Could you check a few things on this model? Use its own coordinates, in mm. Face numbers are marked on the shaded views. A direction names the side the tool comes from. Round coordinates to 2 decimals unless told otherwise and drop trailing zeros. Loops run counter-clockwise (first coordinate to the right, second up) from the corner with the lowest first, then second, coordinate; pieces in that order, holes last. Notation, with made-up numbers: (68.25, -12) -> (125.25, -12) arc R24 ccw to (125.25, 12) -> close; hole circle Ø10 at (68.5, -40). An arc over 180 degrees is marked (long way). One line per item, written item: value.
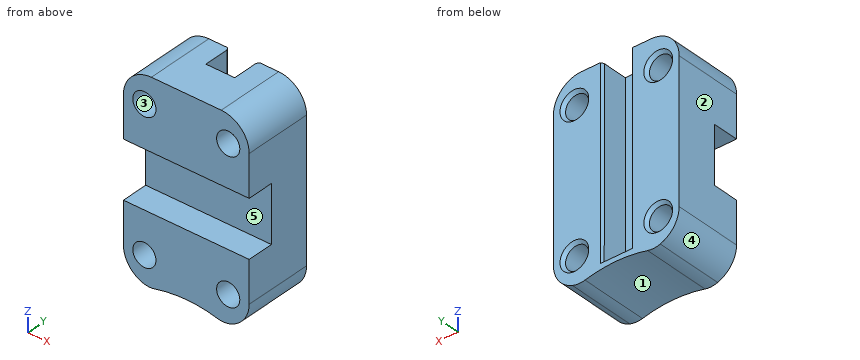
```python
from build123d import *

# Parameters (mm, degrees)
SKETCH1_W               = 45
SKETCH1_H               = 70
BOSS_EXTRUDE1_DEPTH     = 14.5
SKETCH2_W               = 20.25
SKETCH2_H               = 9.5
CUT_EXTRUDE1_DEPTH      = 1
CUT_EXTRUDE1_DEPTH_BACK = 46
SKETCH3_R               = 4.15
CUT_EXTRUDE2_DEPTH      = 15.5
SKETCH5_R               = 4.15
BOSS_EXTRUDE2_DEPTH     = 10
CHAMFER1_SIZE           = 1
CHAMFER1_SIZE2          = 1.191753593
CHAMFER2_SIZE           = 1
CHAMFER2_SIZE2          = 0.577350269
CHAMFER2_PART_2_SIZE    = 1
CHAMFER2_PART_2_SIZE2   = 0.577350269
CHAMFER2_PART_3_SIZE    = 1
CHAMFER2_PART_3_SIZE2   = 0.577350269
FILLET1_R               = 10
CUT_EXTRUDE3_DEPTH      = 25.5
FILLET2_R               = 8


with BuildPart() as part:
    # Sketch1 → Boss-Extrude1 (new body)
    with BuildSketch(Plane(origin=(0, 0, 0), x_dir=(1, 0, 0), z_dir=(0, 1, 0))):
        Rectangle(SKETCH1_W, SKETCH1_H)
    extrude(amount=BOSS_EXTRUDE1_DEPTH)

    # Sketch2 → Cut-Extrude1 (cut, two sides)
    with BuildSketch(Plane(origin=(22.5, 0, 0), x_dir=(0, 0, -1), z_dir=(1, 0, 0))) as cut_extrude1_sk:
        with Locations((0, 4.75)):
            Rectangle(SKETCH2_W, SKETCH2_H)
    extrude(amount=CUT_EXTRUDE1_DEPTH, mode=Mode.SUBTRACT)
    extrude(cut_extrude1_sk.sketch, amount=-CUT_EXTRUDE1_DEPTH_BACK, mode=Mode.SUBTRACT)

    # Sketch3 → Cut-Extrude2 (cut, through all)
    with BuildSketch(Plane.XZ):
        with Locations((15, 25)):
            Circle(SKETCH3_R)
        with Locations((15, -25)):
            Circle(SKETCH3_R)
        with Locations((-15, -25)):
            Circle(SKETCH3_R)
        with Locations((-15, 25)):
            Circle(SKETCH3_R)
    extrude(amount=-CUT_EXTRUDE2_DEPTH, mode=Mode.SUBTRACT)

    # Sketch5 → Boss-Extrude2 (add)
    with BuildSketch(Plane(origin=(0, 14.5, 0), x_dir=(1, 0, 0), z_dir=(0, 1, 0))):
        Polygon((-5.15, -35), (-22.5, -35), (-22.5, 35), (22.5, 35), (22.5, -35), (5.15, -35), (5.130229348, -34.949305848), (5.15, 31), (-5.15, 31), align=None)
        with Locations((-15, 25)):
            Circle(SKETCH5_R, mode=Mode.SUBTRACT)
        with Locations((15, 25)):
            Circle(SKETCH5_R, mode=Mode.SUBTRACT)
        with Locations((15, -25)):
            Circle(SKETCH5_R, mode=Mode.SUBTRACT)
        with Locations((-15, -25)):
            Circle(SKETCH5_R, mode=Mode.SUBTRACT)
    extrude(amount=BOSS_EXTRUDE2_DEPTH)

    # Chamfer1
    chamfer1_edges = [part.edges().sort_by_distance(p)[0] for p in [
        (-19.15, 24.5, -25),
        (10.85, 24.5, -25),
        (10.85, 24.5, 25),
        (-19.15, 24.5, 25),
    ]]
    chamfer1_side = [part.faces().sort_by_distance(p)[0] for p in [
        (-13.825, 24.5, 34.167834151),
    ]]
    chamfer(chamfer1_edges, length=CHAMFER1_SIZE, length2=CHAMFER1_SIZE2, reference=chamfer1_side[0])

    # Chamfer2
    chamfer2_edges = [part.edges().sort_by_distance(p)[0] for p in [
        (-5.15, 24.5, 2),
    ]]
    chamfer2_side = [part.faces().sort_by_distance(p)[0] for p in [
        (-5.15, 19.5, 2),
    ]]
    chamfer(chamfer2_edges, length=CHAMFER2_SIZE, length2=CHAMFER2_SIZE2, reference=chamfer2_side[0])

    # Chamfer2 part 2
    chamfer2_part_2_edges = [part.edges().sort_by_distance(p)[0] for p in [
        (0, 24.5, -31),
    ]]
    chamfer2_part_2_side = [part.faces().sort_by_distance(p)[0] for p in [
        (0, 19.5, -31),
    ]]
    chamfer(chamfer2_part_2_edges, length=CHAMFER2_PART_2_SIZE, length2=CHAMFER2_PART_2_SIZE2, reference=chamfer2_part_2_side[0])

    # Chamfer2 part 3
    chamfer2_part_3_edges = [part.edges().sort_by_distance(p)[0] for p in [
        (5.140114674, 24.5, 1.974652924),
    ]]
    chamfer2_part_3_side = [part.faces().sort_by_distance(p)[0] for p in [
        (5.140114674, 19.5, 1.974652924),
    ]]
    chamfer(chamfer2_part_3_edges, length=CHAMFER2_PART_3_SIZE, length2=CHAMFER2_PART_3_SIZE2, reference=chamfer2_part_3_side[0])

    # Fillet1
    fillet1_edges = [part.edges().sort_by_distance(p)[0] for p in [
        (-22.5, 12.25, -35),
        (22.5, 12.25, -35),
        (22.5, 12.25, 35),
        (-22.5, 12.25, 35),
    ]]
    fillet(fillet1_edges, radius=FILLET1_R)

    # Sketch6 → Cut-Extrude3 (cut, through all)
    with BuildSketch(Plane.XZ):
        with BuildLine():
            Line((12.5, -35), (-12.5, -35))
            ThreePointArc((-12.5, -35), (0, -33.26906369), (12.5, -35))
        make_face()
    extrude(amount=-CUT_EXTRUDE3_DEPTH, mode=Mode.SUBTRACT)

    # Fillet2
    fillet2_edges = [part.edges().sort_by_distance(p)[0] for p in [
        (12.5, 12.25, -35),
        (-12.5, 12.25, -35),
    ]]
    fillet(fillet2_edges, radius=FILLET2_R)


solid = part.part
```
Item 1: If we section it at B-B on x = 2: List the corners of the cut face in (y, z) for me (3 decimals), plus the area to 3 significant figures.
Output:
outline: (0, -33.313) -> (24.5, -33.313) -> (24.5, -31.577) -> (23.5, -31) -> (14.5, -31) -> (14.5, 35) -> (0, 35) -> (0, 10.125) -> (9.5, 10.125) -> (9.5, -10.125) -> (0, -10.125) -> close
area: 821 mm²
Item 2: If we section it at C-C on z = 13.5: List the corners of the cut face in (x, y) for me.
Output:
outline: (-22.5, 0) -> (22.5, 0) -> (22.5, 24.5) -> (5.71, 24.5) -> (5.14, 23.5) -> (5.14, 14.5) -> (-5.15, 14.5) -> (-5.15, 23.5) -> (-5.73, 24.5) -> (-22.5, 24.5) -> close
Item 3: If we section it at A-A on y = 1.5: Count the separate pieces of the cut face and the enclosed holes in it, plus the area to 3 significant figures.
Output:
separate pieces: 2
enclosed holes: 4
area: 1,910 mm²
Item 4: I need wall thicknesses on line 1 (X direction, y = 11, z = 25); line 2 (Z direction, x = 15, y = 7.75) (3 decimals); line 3 (X direction, y = 19, z = 20). Which ranges of each line are inside material? Lowest first, please. Write a range as from..to.
Output:
line 1: x = -22.5..-19.15, -10.85..10.85, 19.15..22.5
line 2: z = -34.675..-29.15, -20.85..-10.125, 10.125..20.85, 29.15..34.682
line 3: x = -22.5..-5.15, 5.13..22.5
Item 5: For the marked faces 4 and 5, which set-ups out of +Z, -Z, +X, -X, +Y, -Y let a thin tool reach every point of the face, with its end or its side?
Output:
face 4: -Z, -X, +Y, -Y
face 5: +X, -X, -Y
Item 6: If we mould it in two halves opening along Z, with no side actions, what happens to the marked faces 1, 2 and 3? For each: released by +Z, released by -Z, zero draft, split by the parting line, or undercut.
Output:
face 1: released by -Z
face 2: zero draft
face 3: undercut
Item 7: Will these pins go through, and if not, where does the flat tip stop? pin 1 Ø1.5 at (x, y) = (3.5, 17.5) entering from -Z; pin 2 Ø6 at (x, z) = (2.5, -1.5) entering from -Y; pin 3 Ø5 at (x, y) = (4.5, 9.5) entering from -Z; pin 4 Ø7.5 at (x, z) = (15, 25) entering from +Y.
Output:
pin 1: stops at z = -33.47
pin 2: stops at y = 9.5
pin 3: stops at z = -33.8
pin 4: passes through
